from build123d import *

# Parameters (mm, degrees)
SKETCH1_W             = 184.15
SKETCH1_H             = 127
BOSS_EXTRUDE1_DEPTH   = 3.175
SKETCH3_R             = 1.35
CUT_EXTRUDE1_DEPTH    = 112.893414686
F_6_CLEARANCE_HOLE1_D = 3.7973
SKETCH9_R             = 1.0999978
CUT_EXTRUDE2_DEPTH    = 112.893414686
SKETCH10_R            = 1.27
CUT_EXTRUDE3_DEPTH    = 112.893414686
SKETCH11_R            = 1.778
CUT_EXTRUDE4_DEPTH    = 112.893414686
SKETCH12_W            = 76.2
SKETCH12_H            = 50.8
CUT_EXTRUDE5_DEPTH    = 112.893414686


with BuildPart() as part:
    # Sketch1 → Boss-Extrude1 (new body)
    with BuildSketch(Plane.XY):
        Rectangle(SKETCH1_W, SKETCH1_H)
    extrude(amount=BOSS_EXTRUDE1_DEPTH)

    # Sketch3 → Cut-Extrude1 (cut, through all)
    with BuildSketch(Plane.XY.offset(3.175)):
        with Locations((-79.800000039, 39.825)):
            Circle(SKETCH3_R)
        with Locations((-21.799999961, 39.825)):
            Circle(SKETCH3_R)
        with Locations((-79.800000039, -46.175)):
            Circle(SKETCH3_R)
        with Locations((-21.799999961, -46.175)):
            Circle(SKETCH3_R)
    extrude(amount=-CUT_EXTRUDE1_DEPTH, mode=Mode.SUBTRACT)

    # #6 Clearance Hole1 (through all)
    with Locations(Plane.XY.offset(3.175)):
        with Locations((-66.675, 53.721), (85.725, 53.721)):
            f_6_clearance_hole1 = Hole(F_6_CLEARANCE_HOLE1_D / 2)

    # Mirror3: #6 Clearance Hole1 across plane
    add(f_6_clearance_hole1.mirror(Plane.ZX), mode=Mode.SUBTRACT)

    # Sketch9 → Cut-Extrude2 (cut, through all)
    with BuildSketch(Plane.XY.offset(3.175)):
        with Locations((18.650000038, -36.45)):
            Circle(SKETCH9_R)
        with Locations((32.149999962, -36.45)):
            Circle(SKETCH9_R)
        with Locations((32.149999962, -52.45)):
            Circle(SKETCH9_R)
        with Locations((18.650000038, -52.45)):
            Circle(SKETCH9_R)
    extrude(amount=-CUT_EXTRUDE2_DEPTH, mode=Mode.SUBTRACT)

    # Sketch10 → Cut-Extrude3 (cut, through all)
    with BuildSketch(Plane.XY.offset(3.175)):
        with Locations((54.61, 46.99)):
            Circle(SKETCH10_R)
        with Locations((54.61, 29.21)):
            Circle(SKETCH10_R)
        with Locations((8.89, 29.21)):
            Circle(SKETCH10_R)
        with Locations((8.89, 46.99)):
            Circle(SKETCH10_R)
    extrude(amount=-CUT_EXTRUDE3_DEPTH, mode=Mode.SUBTRACT)

    # Sketch11 → Cut-Extrude4 (cut, through all)
    with BuildSketch(Plane.XY.offset(3.175)):
        with Locations((57.15, 0)):
            Circle(SKETCH11_R)
        with BuildLine():
            Line((58.928, -46.863), (58.928, -53.213))
            ThreePointArc((58.928, -53.213), (57.15, -54.991), (55.372, -53.213))
            Line((55.372, -53.213), (55.372, -46.863))
            ThreePointArc((55.372, -46.863), (57.15, -45.085), (58.928, -46.863))
        make_face()
    extrude(amount=-CUT_EXTRUDE4_DEPTH, mode=Mode.SUBTRACT)

    # Sketch12 → Cut-Extrude5 (cut, through all)
    with BuildSketch(Plane.XY.offset(3.175)):
        with Locations((-38.1, 0)):
            Rectangle(SKETCH12_W, SKETCH12_H)
    extrude(amount=-CUT_EXTRUDE5_DEPTH, mode=Mode.SUBTRACT)


solid = part.part
Input: part model. Units: mm. Frame: model coordinates. Give positions to 0.01 mm unless a question says otherwise; leave off trailing zeros. Order: outer loops, then holes, each group sorted by start corner. A loop starts at its lowest first (then second) coordinate and runs counter-clockwise, first axis right, second up. Notation, with made-up numbers: (74, 83.25) - (102, 83.25) arc R21 cw to (102, 110.25) - close; hole circle Ø11 at (-4.5, -2). An arc over 180 degrees is marked (long way). Answer as a JSON object with one key per item and string values. Group by question number.
Q1. Line query: probe 1 along Y at (x, z) = (54.61, 2.1); probe 2 along Y at (x, z) = (-62.5, 1.15); probe 3 along X at (y, z) = (-23.5, 2.9) (3 decimals). Output: solid intervals per line, ascending.
Q2. Cut plane A-A, the plane x = -10. Output: boundary loops of the cut face in (y, z) (3 decimals), then the cut area to 3 significant figures.
Q3. First-contact query: pin 1 Ø2.5 at (x, y) = (-21.8, -46.175) entering from +Z. Flat tip, straight axial feed; report the tip coordinate or a pass-through.
Q4. Mould query, pull axis Y, two halves, no side actions, for faces 1 (the face through (19, 1, 0)), 2 (the face through (-68.429, 52.994, 1.565)). Classes: pulls with the +Y half, pulls with the -Y half, needs draft (parallel to the pull), parting line crosses it, or undercut.
Q5. Cut plane B-B, the plane y = -20.5. Output: boundary loops of the cut face in (x, z) (3 decimals).
Q6. Cut plane C-C, the plane z = 1.5. Count the separate pieces of the cut face and the enclosed holes in it, then the cut area to 3 significant figures.
Results:
{
 "1": {"probe 1": "-63.5 to 27.94, 30.48 to 45.72, 48.26 to 63.5", "probe 2": "-63.5 to -25.4, 25.4 to 63.5", "probe 3": "-92.075 to -76.2, 0 to 92.075"},
 "2": {"outline": "(-63.5, 0) - (-25.4, 0) - (-25.4, 3.175) - (-63.5, 3.175) - close; (25.4, 0) - (63.5, 0) - (63.5, 3.175) - (25.4, 3.175) - close", "area": "242 mm^2"},
 "3": {"pin 1": "through"},
 "4": {"face 1": "needs draft", "face 2": "undercut"},
 "5": {"outline": "(-92.075, 0) - (-76.2, 0) - (-76.2, 3.175) - (-92.075, 3.175) - close; (0, 0) - (92.075, 0) - (92.075, 3.175) - (0, 3.175) - close"},
 "6": {"separate pieces": "1", "enclosed holes": "19", "area": "19,400 mm^2"}
}
